Input: part model. Units: mm. Frame: model coordinates. Face numbers are marked on the shaded views. A direction names the side the tool comes from. Give positions to 0.01 mm unless a question says otherwise; leave off trailing zeros. Loops run counter-clockwise (first coordinate to the right, second up) from the corner with the lowest first, then second, coordinate; pieces in that order, holes last. Notation, with made-up numbers: (9.25, 36) -> (26.25, 36) arc R25 ccw to (26.25, 66) -> close; hole circle Ø3 at (72, -24). An arc over 180 degrees is marked (long way). One line per question, with ' | ' between items.
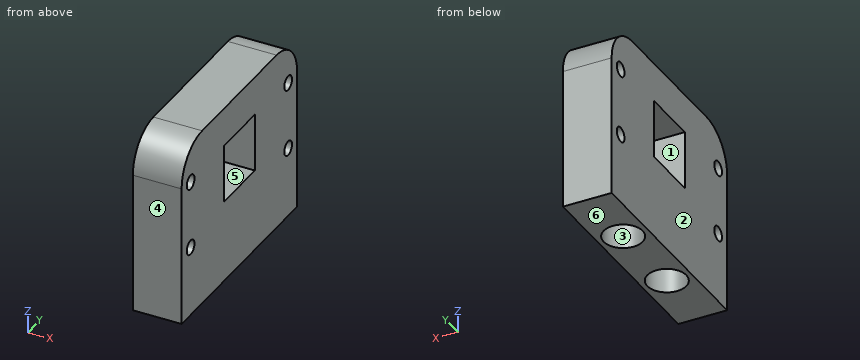
Autodesk Inventor part; units mm, degrees
ref_plane "YZ Plane" through (0, 0, 0) normal (1, 0, 0) x (0, 1, 0)
ref_plane "XZ Plane" through (0, 0, 0) normal (0, 1, 0) x (-1, 0, 0)
ref_plane "XY Plane" through (0, 0, 0) normal (0, 0, 1) x (1, 0, 0)
ref_plane "РабПлоскость1" through (-32.5, 0, 7) normal (-1, 0, 0) x (0, 1, 0)
sketch "Эскиз1" plane through (-32.5, 0, 7) normal (-1, 0, 0) x (0, 1, 0)
  line L0 (15, -5) -> (15, -24)
  arc A0 (15, -5) -> (15, 5) centre (15, 0) ccw
  line L1 (15, -24) -> (-15, -24)
  arc A1 (14.5, -30) -> (22.5, -22) centre (14.5, -22) ccw
  line L2 (-14.5, -30) -> (14.5, -30)
  arc A2 (-22.5, -22) -> (-14.5, -30) centre (-14.5, -22) ccw
  circle A3 centre (-19, -21.5) radius 1.5
  circle A4 centre (-19, -7.5) radius 1.5
  circle A5 centre (19, -21.5) radius 1.5
  circle A6 centre (19, -7.5) radius 1.5
  line L3 (-15, -24) -> (-15, 24) construction
  line L4 (-22.5, 24) -> (-22.5, -22) construction
  line L5 (22.5, -22) -> (22.5, 24) construction
  line L6 (15, 24) -> (15, 5) construction
  line L7 (22.5, -22) -> (22.5, 7)
  line L8 (14, 7) -> (-14, 7)
  line L9 (14, 7) -> (22.5, 7)
  line L10 (-14, 7) -> (-15, 7)
  line L11 (-15, 7) -> (-15, -24)
  line L12 (-22.5, -22) -> (-22.5, 7)
  line L13 (-22.5, 7) -> (-15, 7)
  line L14 (15, 5) -> (15, 7)
  line L15 (-6, -22) -> (6, -22)
  line L16 (6, -22) -> (6, -10)
  line L17 (6, -10) -> (-6, -10)
  line L18 (-6, -10) -> (-6, -22)
  point P0 (0, 7)
  point P1 (0, -10)
  dimension "d0" = 2
  dimension "d1" = 12
  dimension "d2" = 12
extrude "Выдавливание1" add sketch "Эскиз1" along normal blind 10
sketch "Эскиз2" plane through (-32.5, -22.5, 0) normal (0, 0, -1) x (-1, 0, 0)
  arc A0 (7, 34.4641) -> (7, 27.5359) centre (5, 31) ccw
  arc A1 (7, 17.4641) -> (7, 10.5359) centre (5, 14) ccw
  arc A2 (7, 27.5359) -> (7, 34.4641) centre (5, 31) ccw
  arc A3 (7, 10.5359) -> (7, 17.4641) centre (5, 14) ccw
  point P0 (-32.5, 22.5)
extrude "Выдавливание2" cut sketch "Эскиз2" against normal blind 10
equation "\"d2\" = d1"
properties part number "upper_cup"
1. Section query B-B (z = 14.5). Output: boundary loops of the cut face in (x, y).
Determined:
outline: (-42.5, -22.5) -> (-32.5, -22.5) -> (-32.5, -20.5) -> (-42.5, -20.5) -> close; (-42.5, -17.5) -> (-32.5, -17.5) -> (-32.5, 17.5) -> (-42.5, 17.5) -> close; (-42.5, 20.5) -> (-32.5, 20.5) -> (-32.5, 22.5) -> (-42.5, 22.5) -> close
2. Pin query (flat end, axial travel): P1, Ø1.8, axis at y = 19, z = 28.5, coming from the +X side; P2, Ø2.5, axis at x = -37, y = -10, coming from the -Z side. Return the tip coordinate at first contact, or that it passes through.
Determined:
P1: passes through | P2: stops at z = 10
3. Section query C-C (z = 22.5). Output: boundary loops of the cut face in (x, y).
Determined:
outline: (-42.5, -22.5) -> (-32.5, -22.5) -> (-32.5, -6) -> (-42.5, -6) -> close; (-42.5, 6) -> (-32.5, 6) -> (-32.5, 22.5) -> (-42.5, 22.5) -> close
4. Pull-direction query (Z, two-part tool) for the marked faces 4, 5 and 6; classes: pulls with the +Z half, pulls with the -Z half, needs draft (parallel to the pull), parting line crosses it, or undercut.
Determined:
face 4: needs draft | face 5: undercut | face 6: pulls with the -Z half
5. Section query A-A (y = -1.5). Output: boundary loops of the cut face in (x, z).
Determined:
outline: (-42.5, 0) -> (-32.5, 0) -> (-32.5, 17) -> (-42.5, 17) -> close; (-42.5, 29) -> (-32.5, 29) -> (-32.5, 37) -> (-42.5, 37) -> close
6. Ray query, line 1 along Y through (x, z) = (-37.5, 7); line 2 along Y through (x, z) = (-38, 14.5); line 3 along Y through (x, z) = (-39.25, 28.5). Return the intervals inside material, ascending. Write a range as from..to.
Determined:
line 1: y = -22.5..-12.5, -4.5..4.5, 12.5..22.5 | line 2: y = -22.5..-20.5, -17.5..17.5, 20.5..22.5 | line 3: y = -22.5..-20.5, -17.5..-6, 6..17.5, 20.5..22.5
7. Section query D-D (x = -38.5). Output: boundary loops of the cut face in (y, z).
Determined:
outline: (-22.5, 0) -> (-12.37, 0) -> (-12.37, 10) -> (-4.63, 10) -> (-4.63, 0) -> (4.63, 0) -> (4.63, 10) -> (12.37, 10) -> (12.37, 0) -> (22.5, 0) -> (22.5, 29) arc R8 ccw to (14.5, 37) -> (-14.5, 37) arc R8 ccw to (-22.5, 29) -> close; hole circle Ø3 at (-19, 14.5); hole circle Ø3 at (-19, 28.5); hole (-6, 17) -> (6, 17) -> (6, 29) -> (-6, 29) -> close; hole circle Ø3 at (19, 14.5); hole circle Ø3 at (19, 28.5)
8. Reachability of the marked faces 1, 2 and 3 from +Z, -Z, +X, -X, +Y, -Y: full face, straight path, thin tool, end or side. Return the list, or none.
Determined:
face 1: +X, -X | face 2: +Z, -Z, -X, +Y, -Y | face 3: -Z
